```python
from build123d import *

# Parameters (mm, degrees)
SKETCH1_W           = 63.5
SKETCH1_H           = 1.5875
BOSS_EXTRUDE1_DEPTH = 38.1
SKETCH2_R           = 3.175
BOSS_EXTRUDE2_DEPTH = 6.35
SKETCH3_W           = 1.5875
SKETCH3_H           = 18.653125
BOSS_EXTRUDE3_DEPTH = 14.2875


with BuildPart() as part:
    # Sketch1 → Boss-Extrude1 (new body)
    with BuildSketch(Plane.XY):
        with Locations((31.75, 0.79375)):
            Rectangle(SKETCH1_W, SKETCH1_H)
    extrude(amount=BOSS_EXTRUDE1_DEPTH)

    # Sketch2 → Boss-Extrude2 (add)
    with BuildSketch(Plane(origin=(0, 0, 0), x_dir=(-1, 0, 0), z_dir=(0, 0, -1))):
        with BuildLine():
            Line((-38.1, 9.525), (-38.1, 1.5875))
            Line((-38.1, 1.5875), (-25.4, 1.5875))
            Line((-25.4, 1.5875), (-25.4, 9.525))
            Line((-25.4, 9.525), (-25.4, 15.875))
            Line((-25.4, 15.875), (-31.75, 15.875))
            ThreePointArc((-31.75, 15.875), (-36.240128061, 14.015128061), (-38.1, 9.525))
        make_face()
        with Locations((-31.75, 9.525)):
            Circle(SKETCH2_R, mode=Mode.SUBTRACT)
    extrude(amount=-BOSS_EXTRUDE2_DEPTH)

    # Sketch3 → Boss-Extrude3 (add)
    with BuildSketch(Plane(origin=(0, 1.5875, 0), x_dir=(1, 0, 0), z_dir=(0, 1, 0))):
        with Locations((24.60625, -9.3265625)):
            Rectangle(SKETCH3_W, SKETCH3_H)
    extrude(amount=BOSS_EXTRUDE3_DEPTH)


solid = part.part
```
Geometry check sheet. Reference: the model listing, model coordinates, mm. A direction names the side the tool comes from. Give positions to 0.01 mm unless a question says otherwise; leave off trailing zeros. Order: outer loops, then holes, each group sorted by start corner. A loop starts at its lowest first (then second) coordinate and runs counter-clockwise, first axis right, second up. Notation, with made-up numbers: (9, 24.5) - (64, 24.5) arc R12 cw to (64, 33.5) - close; hole circle Ø2 at (27.25, -10). An arc over 180 degrees is marked (long way). Answer in a Markdown table with one row per item. Add a question column.
Q1. Cross-section at C-C, the plane y = 2.75. Enter the section's corners in (x, z).
Q2. Cross-section at B-B, the plane z = 16. Enter the section's corners in (x, y) (1 decimal).
Q3. Tool access check on faces 4 (the flat face through (31, 1, 38.1)), 5 (the flat face through (23.812, 9, 9)), 6 (the flat face through (32, 6, 6.35)), 7 (the flat face through (38.1, 6, 3)), 8 (the flat face through (25, 9, 18.653)). Record the directions out of +Z, -Z, +X, -X, +Y, -Y that give a thin tool (end or side, any length) a straight path to the whole face; none if there is none.
Q4. Gauge pin test, flat ends, axial feed: pin 1 (1 mm diameter, centred on x = 18, y = 3, fed in from -Z); pin 2 (1.9 mm diameter, centred on y = 6.5, z = 4, fed in from +X); pin 3 (8 mm diameter, centred on x = 23.5, z = 22.5, fed in from +Y) (3 decimals); pin 4 (8.5 mm diameter, centred on x = 31.75, y = 9.525, fed in from +Z). Record the tip position at first contact, or that the pin passes through.
Q5. Material ranges on probe 1 along Y at (x, z) = (31.75, 4) (3 decimals); probe 2 along X at (y, z) = (7.75, 13.5); probe 3 along Y at (x, z) = (55, 20), recorded low to high. Write a range as from..to.
Q6. Cross-section at A-A, the plane y = 11. Enter the section's corners in (x, z), then the cut area to 3 significant figures.
Q7. Mould release check, pull along X, two halves, no side actions. Record for faces 1 (the cylindrical face through (34.09, 11.67, 3.13)), 2 (the flat face through (0, 1, 19)), 3 (the flat face through (25.4, 9, 13)): pulls with the +X half, pulls with the -X half, needs draft (parallel to the pull), parting line crosses it, or undercut.
Q8. Cross-section at D-D, the plane x = 9.5. Enter the section's corners in (y, z), then the cut area to 3 significant figures.
Check values:
| question | item | result |
|---|---|---|
| 1 | outline | (23.81, 0) - (38.1, 0) - (38.1, 6.35) - (25.4, 6.35) - (25.4, 18.65) - (23.81, 18.65) - close |
| 2 | outline | (0, 0) - (63.5, 0) - (63.5, 1.6) - (25.4, 1.6) - (25.4, 15.9) - (23.8, 15.9) - (23.8, 1.6) - (0, 1.6) - close |
| 3 | face 4 | +Z, +X, -X, +Y, -Y |
| 3 | face 5 | +Z, -Z, -X, +Y |
| 3 | face 6 | +Z, +X, +Y |
| 3 | face 7 | +Z, -Z, +X, +Y |
| 3 | face 8 | +Z, +X, -X, +Y |
| 4 | pin 1 | passes through |
| 4 | pin 2 | stops at x = 38.1 |
| 4 | pin 3 | stops at y = 15.875 |
| 4 | pin 4 | stops at z = 6.35 |
| 5 | probe 1 | y = 0..6.35, 12.7..15.875 |
| 5 | probe 2 | x = 23.81..25.4 |
| 5 | probe 3 | y = 0..1.59 |
| 6 | outline | (23.81, 0) - (28.94, 0) - (28.94, 6.35) - (25.4, 6.35) - (25.4, 18.65) - (23.81, 18.65) - close; (34.56, 0) - (37.93, 0) - (37.93, 6.35) - (34.56, 6.35) - close |
| 6 | area | 73.4 mm^2 |
| 7 | face 1 | undercut |
| 7 | face 2 | pulls with the -X half |
| 7 | face 3 | pulls with the +X half |
| 8 | outline | (0, 0) - (1.59, 0) - (1.59, 38.1) - (0, 38.1) - close |
| 8 | area | 60.5 mm^2 |
